Autodesk Inventor part; units mm, degrees
ref_plane "YZ Plane" through (0, 0, 0) normal (1, 0, 0) x (0, 1, 0)
ref_plane "XZ Plane" through (0, 0, 0) normal (0, 1, 0) x (-1, 0, 0)
ref_plane "XY Plane" through (0, 0, 0) normal (0, 0, 1) x (1, 0, 0)
sketch "Sketch1" plane through (0, 0, 0) normal (0, 0, 1) x (1, 0, 0)
  line L0 (0, 0) -> (88.9, 0)
  line L1 (88.9, 0) -> (88.9, 6.35)
  line L2 (88.9, 6.35) -> (6.35, 6.35)
  line L3 (6.35, 6.35) -> (6.35, 44.45)
  line L4 (6.35, 44.45) -> (6.35, 127)
  line L5 (6.35, 127) -> (0, 127)
  line L6 (0, 127) -> (0, 0)
  dimension "d0" = 88.9
  dimension "d1" = 127
  dimension "d2" = 6.35
extrude "Extrusion1" add sketch "Sketch1" along normal blind 63.5
sketch "Sketch2" plane through (6.35, 6.35, 0) normal (0, 1, 0) x (1, 0, 0)
  line L0 (67.55, -51) -> (15, -51) construction
  line L1 (15, -51) -> (15, -12.5) construction
  line L2 (15, -12.5) -> (67.55, -12.5) construction
  line L3 (67.55, -12.5) -> (67.55, -51) construction
  circle A0 centre (67.55, -51) radius 3.175
  circle A1 centre (67.55, -12.5) radius 3.175
  circle A2 centre (41.275, -51) radius 3.175
  circle A3 centre (41.275, -12.5) radius 3.175
  circle A4 centre (15, -51) radius 3.175
  circle A5 centre (15, -12.5) radius 3.175
  line L4 (0, 0) -> (82.55, 0) construction
  line L5 (82.55, 0) -> (82.55, -63.5) construction
  line L6 (82.55, -63.5) -> (0, -63.5) construction
  line L7 (0, -63.5) -> (0, 0) construction
  line L8 (67.55, -31.75) -> (82.55, -31.75) construction
  line L9 (15, -31.75) -> (0, -31.75) construction
  point P0 (-6.35, 0)
  dimension "d5" = 6.35
  dimension "d6" = 6.35
  dimension "d7" = 63.5
  dimension "d9" = 88.9
  dimension "d10" = 15
  dimension "d11" = 12.5
extrude "Extrusion2" cut sketch "Sketch2" against normal through all
properties part number "L_Channel" material "Steel, Mild"
Could you check a few things on this model? Use its own coordinates, in mm. A direction names the side the tool comes from. Give positions to 0.01 mm unless a question says otherwise; leave off trailing zeros. Loops run counter-clockwise (first coordinate to the right, second up) from the corner with the lowest first, then second, coordinate; pieces in that order, holes last. Notation, with made-up numbers: M 44.25,-34 L 82.25,-34 A31 ccw 82.25,5 Z; hole C -28,3 d4. An arc over 180 degrees is marked long. Answer as a JSON object with one key per item and string values.
Q1. Suppose I cut it at A-A, the plane z = 51. List the corners of the cut face in (x, y) for me (3 decimals).
Values found:
{"outline": "M 0,0 L 18.175,0 L 18.175,6.35 L 6.35,6.35 L 6.35,127 L 0,127 Z; M 24.525,0 L 44.45,0 L 44.45,6.35 L 24.525,6.35 Z; M 50.8,0 L 70.725,0 L 70.725,6.35 L 50.8,6.35 Z; M 77.075,0 L 88.9,0 L 88.9,6.35 L 77.075,6.35 Z"}
Q2. For faces 5 (the flat face through (44, 0, 31)), 6 (the flat face through (48, 6.35, 31)), which set-ups out of +Z, -Z, +X, -X, +Y, -Y let a thin tool reach every point of the face, with its end or its side?
Values found:
{"face 5": "+Z, -Z, +X, -X, -Y", "face 6": "+Z, -Z, +X, +Y"}
Q3. Suppose I cut it at C-C, the plane y = 9. List the corners of the cut face in (x, z) for me.
Values found:
{"outline": "M 0,0 L 6.35,0 L 6.35,63.5 L 0,63.5 Z"}
Q4. If I drill on probe 1 along X at (y, z) = (2, 51) (3 decimals); probe 2 along X at (y, z) = (60.5, 55), over which ranges is the centre line in solid material (lowest first)? Write a range as [from, to].
Values found:
{"probe 1": "x = [0, 18.175], [24.525, 44.45], [50.8, 70.725], [77.075, 88.9]", "probe 2": "x = [0, 6.35]"}
Q5. If we mould it in two halves opening along Z, with no side actions, what happens to faces 1 (the cylindrical face through (50.558, 3.219, 13.716)), 2 (the flat face through (5, 45, 0)), 3 (the flat face through (6.35, 66, 31)), 4 (the flat face through (5, 45, 63.5))? For each: pulls with the +Z half, pulls with the -Z half, needs draft (parallel to the pull), parting line crosses it, or undercut.
Values found:
{"face 1": "undercut", "face 2": "pulls with the -Z half", "face 3": "needs draft", "face 4": "pulls with the +Z half"}
Q6. Suppose I cut it at B-B, the plane x = 22. List the corners of the cut face in (y, z) for me.
Values found:
{"outline": "M 0,0 L 6.35,0 L 6.35,9.39 L 0,9.39 Z; M 0,15.61 L 6.35,15.61 L 6.35,47.89 L 0,47.89 Z; M 0,54.11 L 6.35,54.11 L 6.35,63.5 L 0,63.5 Z"}
Q7. For P1, Ø5, axis at x = 33.5, z = 20.5, coming from the +Y side; P2, Ø3, axis at y = 88.5, z = 13, coming from the +X side, each with a flat end and sliding along its axis, tell me the tip position at first contact or that it passes through.
Values found:
{"P1": "stops at y = 6.35", "P2": "stops at x = 6.35"}
Q8. Suppose I cut it at D-D, the plane z = 19.5. List the corners of the cut face in (x, y) for me, plus the area to 3 significant figures.
Values found:
{"outline": "M 0,0 L 88.9,0 L 88.9,6.35 L 6.35,6.35 L 6.35,127 L 0,127 Z", "area": "1,330 mm²"}
